Check sheet for the drawn part. Datum: minimum x, y, z corner. Units: mm. A direction names the side the tool comes from. Coordinates: 2 decimals unless noted, no trailing zeros. Order: outer loops, then holes, each group sorted by start corner. A loop starts at its lowest first (then second) coordinate and runs counter-clockwise, first axis right, second up. Notation, with made-up numbers: (6, 64.5) - (13, 64.5) arc R22 cw to (13, 84.5) - close; hole circle Ø11 at (59, 10). An arc over 180 degrees is marked (long way). Return JSON: item names as keys, results as strings. Group by question number.
Item 1: Draft check along X on the marked faces 1, 2 and 3. Enter one of: pulls with the +X half, pulls with the -X half, needs draft (parallel to the pull), parting line crosses it, or undercut.
Item 2: Section check A-A on y = 17.25. Enter the section's corners in (x, z), then the cut area to 3 significant figures.
Item 3: Gauge pin test, flat ends, axial feed: pin 1 (1.5 mm diameter, centred on x = 5, y = 11, fed in from +Z); pin 2 (2 mm diameter, centred on x = 2, y = 13.5, fed in from +Z); pin 3 (0.8 mm diameter, centred on x = 4.5, z = 4, fed in from +Y); pin 4 (1 mm diameter, centred on x = 6, z = 5.5, fed in from -Y). Record the tip position at first contact, or that the pin passes through.
Item 4: Tool access check on the marked faces 4 and 5. Record the directions out of +Z, -Z, +X, -X, +Y, -Y that give a thin tool (end or side, any length) a straight path to the whole face; none if there is none.
Item 5: Scan lines: probe 1 along Y at (x, z) = (6, 5.5); probe 2 along Z at (x, y) = (3.5, 12); probe 3 along X at (y, z) = (10, 3.25). Record each from-to range of solid material in increasing order.
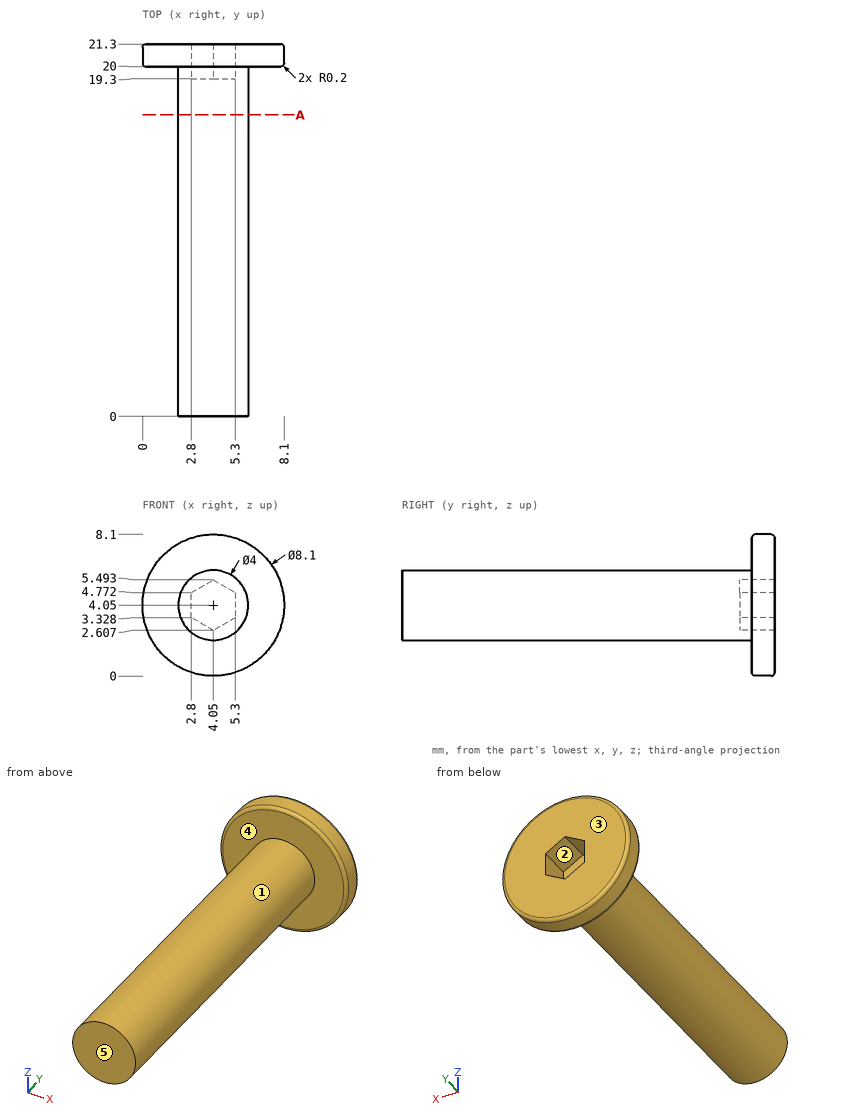
Computed:
{
 "1": {"face 1": "parting line crosses it", "face 2": "undercut", "face 3": "needs draft"},
 "2": {"outline": "circle Ø4 at (4.05, 4.05)", "area": "12.6 mm²"},
 "3": {"pin 1": "stops at z = 6.04", "pin 2": "stops at z = 5.75", "pin 3": "stops at y = 19.3", "pin 4": "stops at y = 0"},
 "4": {"face 4": "-Y", "face 5": "+Z, -Z, +X, -X, -Y"},
 "5": {"probe 1": "y = 20 to 21.3", "probe 2": "z = 2.13 to 5.97", "probe 3": "x = 2.22 to 5.88"}
}
